Source: CAD feature listing. Evaluate the final solid. Frame: model axes, mm. Face numbers are marked on the shaded views. A direction names the side the tool comes from. Round coordinates to 2 decimals unless told otherwise and drop trailing zeros. Order: outer loops, then holes, each group sorted by start corner. A loop starts at its lowest first (then second) coordinate and runs counter-clockwise, first axis right, second up. Notation, with made-up numbers: (-11, 47) -> (19, 47) arc R14 ccw to (19, 55) -> close; hole circle Ø1 at (-20.75, -6.75). An arc over 180 degrees is marked (long way). Answer as CSV lines item,"result". Start each with the question number.
(1) Line query: line 1 along Y through (x, z) = (0, 4.75) (3 decimals); line 2 along Y through (x, z) = (0, 8.9) (3 decimals); line 3 along Z through (x, y) = (-13, -4). Output: solid intervals per line, ascending. Write a range as from..to.
(2) Contact query for flat-ended pins moving along their axis: P1, Ø4, axis at y = -6.5, z = 5, coming from the +X side; P2, Ø10, axis at x = -10, y = -8.5, coming from the -Z side; P3, Ø3, axis at y = -10, z = 4, coming from the +X side; P4, Ø1.5, axis at x = -1, z = 1, coming from the +Y side. Output: stop coordinate, or through.
(3) Section query D-D (x = -9). Output: boundary loops of the cut face in (y, z).
(4) Set-up query: the marked faces 1 and 2. Return all of +Z, -Z, +X, -X, +Y, -Y with unobstructed straight access to the full face (end or side cutting, diameter ignored); none if empty.
(5) Section query A-A (x = 0). Output: boundary loops of the cut face in (y, z) (3 decimals), plus the area to 3 significant figures.
(6) Section query B-B (y = 0). Output: boundary loops of the cut face in (x, z) (1 decimal), plus the area to 3 significant figures.
(7) Pull-direction query (X, two-part tool) for the marked faces 3, 4 and 5; classes: +X half, -X half, draft (parallel to the pull), parting line (faces both ways), or undercut.
```python
from build123d import *

# Parameters (mm, degrees)
BOSS_EXTRUDE1_DEPTH     = 10.16
CUT_EXTRUDE1_DEPTH      = 7.62
CUT_EXTRUDE2_DEPTH      = 33.349183626
CUT_EXTRUDE2_DEPTH_BACK = 33.349183626
SKETCH3_R               = 3.96875
SKETCH3_R_2             = 2.38125


with BuildPart() as part:
    # Sketch1 → Boss-Extrude1 (new body)
    with BuildSketch(Plane.XY):
        with BuildLine():
            Line((8.104909091, 15.108324647), (21.665045455, 7.833946113))
            ThreePointArc((21.665045455, 7.833946113), (26.3525, 0), (21.665045455, -7.833946113))
            Line((21.665045455, -7.833946113), (8.104909091, -15.108324647))
            ThreePointArc((8.104909091, -15.108324647), (-17.145, 0), (8.104909091, 15.108324647))
        make_face()
    extrude(amount=BOSS_EXTRUDE1_DEPTH)

    # Sketch2 → Cut-Extrude1 (cut)
    with BuildSketch(Plane.XY):
        with BuildLine():
            Line((6.904181818, 12.870054329), (20.464318182, 5.595675795))
            ThreePointArc((20.464318182, 5.595675795), (23.8125, 0), (20.464318182, -5.595675795))
            Line((20.464318182, -5.595675795), (6.904181818, -12.870054329))
            ThreePointArc((6.904181818, -12.870054329), (-14.605, 0), (6.904181818, 12.870054329))
        make_face()
    extrude(amount=CUT_EXTRUDE1_DEPTH, mode=Mode.SUBTRACT)

    # Sketch3 → Cut-Extrude2 (cut, two sides: drawn at the far end of the back side and taken through both)
    with BuildSketch(Plane(origin=(0, 0, 7.62), x_dir=(-1, 0, 0), z_dir=(0, 0, -1)).offset(-CUT_EXTRUDE2_DEPTH_BACK)):
        Circle(SKETCH3_R)
        with Locations((-17.4625, 0)):
            Circle(SKETCH3_R_2)
    extrude(amount=CUT_EXTRUDE2_DEPTH + CUT_EXTRUDE2_DEPTH_BACK, mode=Mode.SUBTRACT)


solid = part.part
```
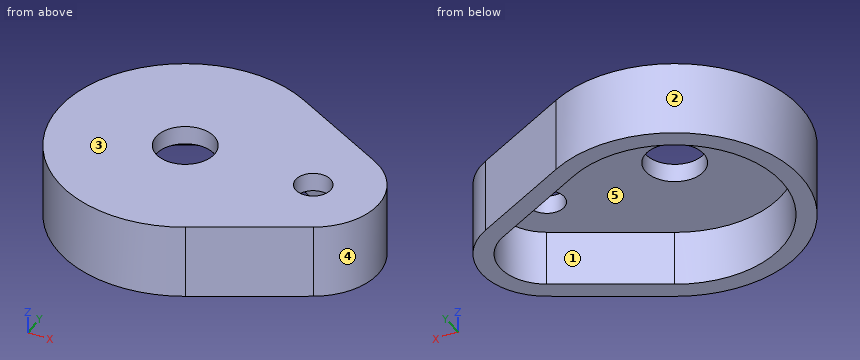
Answer block:
1,line 1,"-17.145..-14.605, 14.605..17.145"
1,line 2,"-17.145..-3.969, 3.969..17.145"
1,line 3,"7.62..10.16"
2,P1,"x = 25.13"
2,P2,"z = 0"
2,P3,"x = 20.42"
2,P4,"y = 17.14"
3,outline,"(-14.59, 0) -> (-11.5, 0) -> (-11.5, 7.62) -> (11.5, 7.62) -> (11.5, 0) -> (14.59, 0) -> (14.59, 10.16) -> (-14.59, 10.16) -> close"
4,face 1,"-Z"
4,face 2,"+Z, -Z"
5,outline,"(-17.145, 0) -> (-14.605, 0) -> (-14.605, 7.62) -> (-3.969, 7.62) -> (-3.969, 10.16) -> (-17.145, 10.16) -> close; (3.969, 7.62) -> (14.605, 7.62) -> (14.605, 0) -> (17.145, 0) -> (17.145, 10.16) -> (3.969, 10.16) -> close"
5,area,"106 mm2"
6,outline,"(-17.1, 0) -> (-14.6, 0) -> (-14.6, 7.6) -> (-4, 7.6) -> (-4, 10.2) -> (-17.1, 10.2) -> close; (4, 7.6) -> (15.1, 7.6) -> (15.1, 10.2) -> (4, 10.2) -> close; (19.8, 7.6) -> (23.8, 7.6) -> (23.8, 0) -> (26.4, 0) -> (26.4, 10.2) -> (19.8, 10.2) -> close"
6,area,"117 mm2"
7,face 3,"draft"
7,face 4,"+X half"
7,face 5,"undercut"
